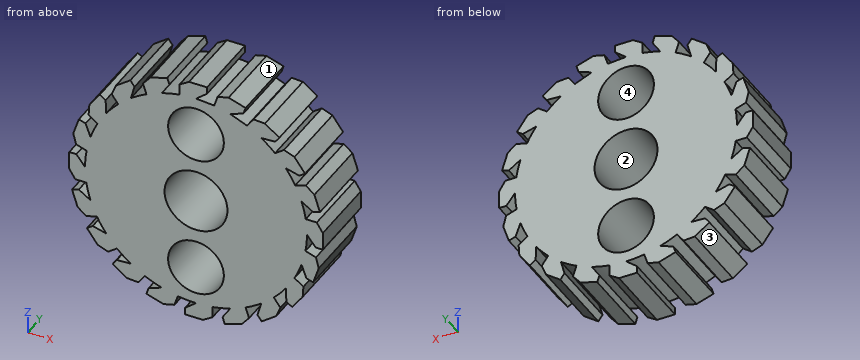
```python
from build123d import *

# Parameters (mm, degrees)
F0_R     = 9.675
F0_R_2   = 10.925
F1_DEPTH = 25


with BuildPart() as f1:
    # F0 (on Front) → F1 (new body)
    with BuildSketch(Plane.XZ):
        with BuildLine():
            Line((3.806459, 44), (-2.426446, 44))
            Line((-2.426446, 44), (-5.736627, 41.90996))
            Line((-5.736627, 41.90996), (-5.736627, 38.070213))
            ThreePointArc((-5.736627, 38.070213), (-8.846834, 37.469768), (-11.897154, 36.615676))
            Line((-11.897154, 36.615676), (-9.217365, 40.686093))
            Line((-9.217365, 40.686093), (-9.97659, 43.022747))
            Line((-9.97659, 43.022747), (-15.904435, 41.096674))
            Line((-15.904435, 41.096674), (-18.406746, 38.086026))
            Line((-18.406746, 38.086026), (-17.220199, 34.434209))
            ThreePointArc((-17.220199, 34.434209), (-19.992635, 32.902045), (-22.629732, 31.147154))
            Line((-22.629732, 31.147154), (-21.338929, 35.846452))
            Line((-21.338929, 35.846452), (-22.783061, 37.834129))
            Line((-22.783061, 37.834129), (-27.825587, 34.170519))
            Line((-27.825587, 34.170519), (-29.275085, 30.533966))
            Line((-29.275085, 30.533966), (-27.018138, 27.427545))
            ThreePointArc((-27.018138, 27.427545), (-29.181416, 25.11364), (-31.147154, 22.629732))
            Line((-31.147154, 22.629732), (-31.37169, 27.49791))
            Line((-31.37169, 27.49791), (-33.359367, 28.942042))
            Line((-33.359367, 28.942042), (-37.022977, 23.899515))
            Line((-37.022977, 23.899515), (-37.277775, 19.993028))
            Line((-37.277775, 19.993028), (-34.171354, 17.736081))
            ThreePointArc((-34.171354, 17.736081), (-35.513718, 14.866938), (-36.615676, 11.897154))
            Line((-36.615676, 11.897154), (-38.333572, 16.457681))
            Line((-38.333572, 16.457681), (-40.670226, 17.216906))
            Line((-40.670226, 17.216906), (-42.5963, 11.289061))
            Line((-42.5963, 11.289061), (-41.631456, 7.495034))
            Line((-41.631456, 7.495034), (-37.979639, 6.308487))
            ThreePointArc((-37.979639, 6.308487), (-38.369689, 3.164956), (-38.5, 0))
            Line((-38.5, 0), (-41.543096, 3.806459))
            Line((-41.543096, 3.806459), (-44, 3.806459))
            Line((-44, 3.806459), (-44, -2.426446))
            Line((-44, -2.426446), (-41.90996, -5.736627))
            Line((-41.90996, -5.736627), (-38.070213, -5.736627))
            ThreePointArc((-38.070213, -5.736627), (-37.469768, -8.846834), (-36.615676, -11.897154))
            Line((-36.615676, -11.897154), (-40.686093, -9.217365))
            Line((-40.686093, -9.217365), (-43.022747, -9.97659))
            Line((-43.022747, -9.97659), (-41.096674, -15.904435))
            Line((-41.096674, -15.904435), (-38.086026, -18.406746))
            Line((-38.086026, -18.406746), (-34.434209, -17.220199))
            ThreePointArc((-34.434209, -17.220199), (-32.902045, -19.992635), (-31.147154, -22.629732))
            Line((-31.147154, -22.629732), (-35.846452, -21.338929))
            Line((-35.846452, -21.338929), (-37.834129, -22.783061))
            Line((-37.834129, -22.783061), (-34.170519, -27.825587))
            Line((-34.170519, -27.825587), (-30.533966, -29.275085))
            Line((-30.533966, -29.275085), (-27.427545, -27.018138))
            ThreePointArc((-27.427545, -27.018138), (-25.11364, -29.181416), (-22.629732, -31.147154))
            Line((-22.629732, -31.147154), (-27.49791, -31.37169))
            Line((-27.49791, -31.37169), (-28.942042, -33.359367))
            Line((-28.942042, -33.359367), (-23.899515, -37.022977))
            Line((-23.899515, -37.022977), (-19.993028, -37.277775))
            Line((-19.993028, -37.277775), (-17.736081, -34.171354))
            ThreePointArc((-17.736081, -34.171354), (-14.866938, -35.513718), (-11.897154, -36.615676))
            Line((-11.897154, -36.615676), (-16.457681, -38.333572))
            Line((-16.457681, -38.333572), (-17.216906, -40.670226))
            Line((-17.216906, -40.670226), (-11.289061, -42.5963))
            Line((-11.289061, -42.5963), (-7.495034, -41.631456))
            Line((-7.495034, -41.631456), (-6.308487, -37.979639))
            ThreePointArc((-6.308487, -37.979639), (-3.164956, -38.369689), (0, -38.5))
            Line((0, -38.5), (-3.806459, -41.543096))
            Line((-3.806459, -41.543096), (-3.806459, -44))
            Line((-3.806459, -44), (2.426446, -44))
            Line((2.426446, -44), (5.736627, -41.90996))
            Line((5.736627, -41.90996), (5.736627, -38.070213))
            ThreePointArc((5.736627, -38.070213), (8.846834, -37.469768), (11.897154, -36.615676))
            Line((11.897154, -36.615676), (9.217365, -40.686093))
            Line((9.217365, -40.686093), (9.97659, -43.022747))
            Line((9.97659, -43.022747), (15.904435, -41.096674))
            Line((15.904435, -41.096674), (18.406746, -38.086026))
            Line((18.406746, -38.086026), (17.220199, -34.434209))
            ThreePointArc((17.220199, -34.434209), (19.992635, -32.902045), (22.629732, -31.147154))
            Line((22.629732, -31.147154), (21.338929, -35.846452))
            Line((21.338929, -35.846452), (22.783061, -37.834129))
            Line((22.783061, -37.834129), (27.825587, -34.170519))
            Line((27.825587, -34.170519), (29.275085, -30.533966))
            Line((29.275085, -30.533966), (27.018138, -27.427545))
            ThreePointArc((27.018138, -27.427545), (29.181416, -25.11364), (31.147154, -22.629732))
            Line((31.147154, -22.629732), (31.37169, -27.49791))
            Line((31.37169, -27.49791), (33.359367, -28.942042))
            Line((33.359367, -28.942042), (37.022977, -23.899515))
            Line((37.022977, -23.899515), (37.277775, -19.993028))
            Line((37.277775, -19.993028), (34.171354, -17.736081))
            ThreePointArc((34.171354, -17.736081), (35.513718, -14.866938), (36.615676, -11.897154))
            Line((36.615676, -11.897154), (38.333572, -16.457681))
            Line((38.333572, -16.457681), (40.670226, -17.216906))
            Line((40.670226, -17.216906), (42.5963, -11.289061))
            Line((42.5963, -11.289061), (41.631456, -7.495034))
            Line((41.631456, -7.495034), (37.979639, -6.308487))
            ThreePointArc((37.979639, -6.308487), (38.369689, -3.164956), (38.5, 0))
            Line((38.5, 0), (41.543096, -3.806459))
            Line((41.543096, -3.806459), (44, -3.806459))
            Line((44, -3.806459), (44, 2.426446))
            Line((44, 2.426446), (41.90996, 5.736627))
            Line((41.90996, 5.736627), (38.070213, 5.736627))
            ThreePointArc((38.070213, 5.736627), (37.469768, 8.846834), (36.615676, 11.897154))
            Line((36.615676, 11.897154), (40.686093, 9.217365))
            Line((40.686093, 9.217365), (43.022747, 9.97659))
            Line((43.022747, 9.97659), (41.096674, 15.904435))
            Line((41.096674, 15.904435), (38.086026, 18.406746))
            Line((38.086026, 18.406746), (34.434209, 17.220199))
            ThreePointArc((34.434209, 17.220199), (32.902045, 19.992635), (31.147154, 22.629732))
            Line((31.147154, 22.629732), (35.846452, 21.338929))
            Line((35.846452, 21.338929), (37.834129, 22.783061))
            Line((37.834129, 22.783061), (34.170519, 27.825587))
            Line((34.170519, 27.825587), (30.533966, 29.275085))
            Line((30.533966, 29.275085), (27.427545, 27.018138))
            ThreePointArc((27.427545, 27.018138), (25.11364, 29.181416), (22.629732, 31.147154))
            Line((22.629732, 31.147154), (27.49791, 31.37169))
            Line((27.49791, 31.37169), (28.942042, 33.359367))
            Line((28.942042, 33.359367), (23.899515, 37.022977))
            Line((23.899515, 37.022977), (19.993028, 37.277775))
            Line((19.993028, 37.277775), (17.736081, 34.171354))
            Line((17.736081, 34.171354), (11.897154, 36.615676))
            Line((11.897154, 36.615676), (16.457681, 38.333572))
            Line((16.457681, 38.333572), (17.216906, 40.670226))
            Line((17.216906, 40.670226), (11.289061, 42.5963))
            Line((11.289061, 42.5963), (7.495034, 41.631456))
            Line((7.495034, 41.631456), (6.308487, 37.979639))
            Line((6.308487, 37.979639), (0, 38.5))
            Line((0, 38.5), (3.806459, 41.543096))
            Line((3.806459, 41.543096), (3.806459, 44))
        make_face()
        with Locations((0, -25)):
            Circle(F0_R, mode=Mode.SUBTRACT)
        Circle(F0_R_2, mode=Mode.SUBTRACT)
        with Locations((0, 25)):
            Circle(F0_R, mode=Mode.SUBTRACT)
    extrude(amount=F1_DEPTH)


solid = f1.part
```
Input: part model. Units: mm. Frame: model coordinates. Face numbers are marked on the shaded views. Round coordinates to 2 decimals unless told otherwise and drop trailing zeros. Loops run counter-clockwise (first coordinate to the right, second up) from the corner with the lowest first, then second, coordinate; pieces in that order, holes last.
1) Section query A-A on x = -25.5. Return the cut outline in (y, z), plus the area to 3 significant figures.
Ans:
outline: (-25, -35.86) - (0, -35.86) - (0, -31.28) - (-25, -31.28) - close; (-25, -28.84) - (0, -28.84) - (0, 35.86) - (-25, 35.86) - close
area: 1,730 mm2
2) Section query D-D on x = 14. Return the cut outline in (y, z), plus the area to 3 significant figures.
Ans:
outline: (-25, -41.72) - (0, -41.72) - (0, 35.74) - (-25, 35.74) - close; (-25, 37.41) - (0, 37.41) - (0, 41.72) - (-25, 41.72) - close
area: 2,040 mm2
3) Material intervals for line 1 (X direction, y = -7.5, z = 40); line 2 (X direction, y = -11.5, z = -32); line 3 (X direction, y = -22, z = -9), sorted ascending.
Ans:
line 1: x = -16.82 to -9.67, -5.74 to 1.88, 6.96 to 17
line 2: x = -27.95 to -6.68, 6.68 to 21.41, 22.4 to 28.69
line 3: x = -37.43 to -6.19, 6.19 to 42.01
4) Section query C-C on y = -21. Count the separate pieces of the cut face and the enclosed holes in it, plus the area to 3 significant figures.
Ans:
separate pieces: 1
enclosed holes: 3
area: 4,570 mm2
5) Section query B-B on z = 25. Return the cut outline in (x, y) (3 decimals).
Ans:
outline: (-36.223, -25) - (-31.256, -25) - (-31.256, 0) - (-36.223, 0) - close; (-29.279, -25) - (-9.675, -25) - (-9.675, 0) - (-29.279, 0) - close; (9.675, -25) - (36.223, -25) - (36.223, 0) - (9.675, 0) - close
6) Pull-direction query (Z, two-part tool) for the marked faces 1, 2, 3 and 4; classes: released by +Z, released by -Z, zero draft, split by the parting line, or undercut.
Ans:
face 1: released by +Z
face 2: undercut
face 3: released by -Z
face 4: undercut
7) Pin query (flat end, axial travel): pin 1 (4 mm diameter, centred on x = 39.5, y = -7, fed in from +Z); pin 2 (3 mm diameter, centred on x = -39, y = -11.5, fed in from -Z); pin 3 (0.7 mm diameter, centred on y = -6.5, z = 43, fed in from +X). Return the tip coordinate at first contact, or that it passes through.
Ans:
pin 1: stops at z = 23.24
pin 2: stops at z = -23.24
pin 3: stops at x = 3.81
